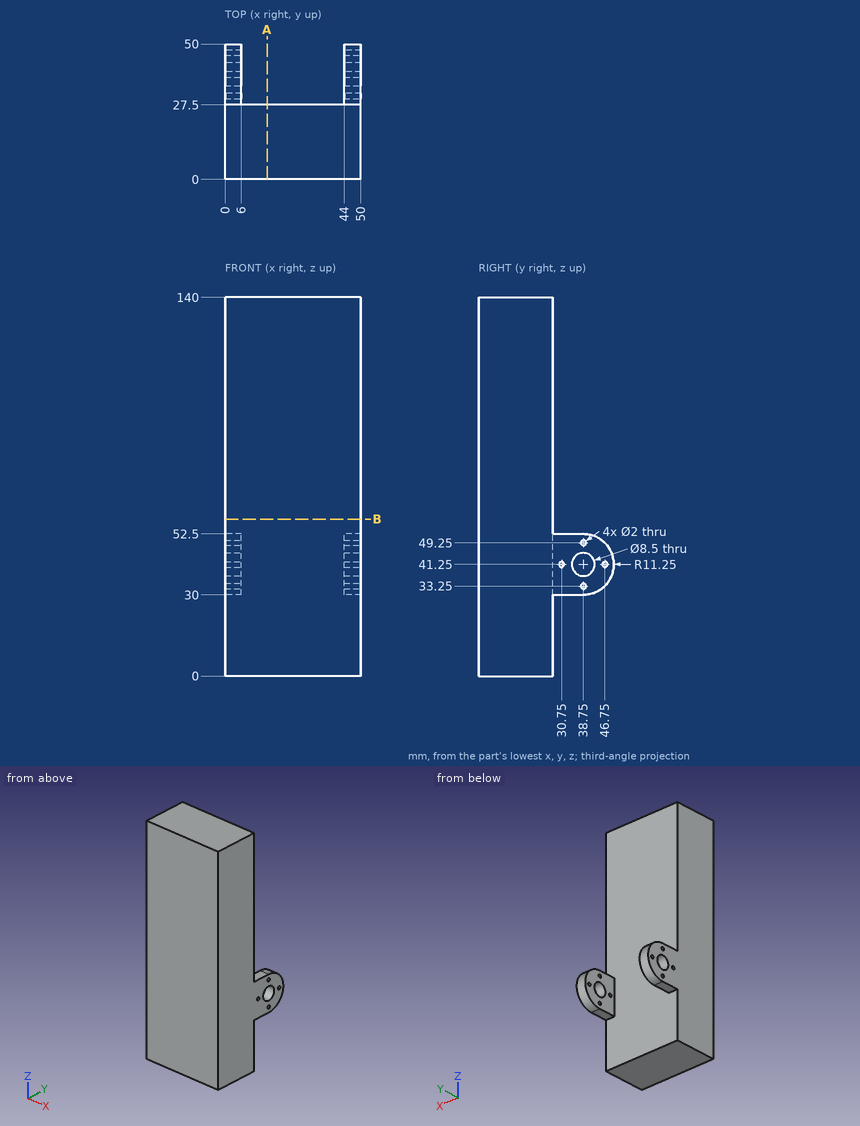
Design review of the part shown in the three views and the two pictorial views. Dimensions are in mm from the part's minimum x, y and z. Round coordinates to 2 decimals unless told otherwise and drop trailing zeros. Loops run counter-clockwise (first coordinate to the right, second up) from the corner with the lowest first, then second, coordinate; pieces in that order, holes last.
(1) Clearance check with flat-ended pins moving along their axes: P1, Ø3, axis at x = 3.5, y = 32.5, coming from the -Z side; P2, Ø3, axis at x = 4, y = 32.5, coming from the +Z side; P3, Ø4, axis at x = 30.5, z = 47.5, coming from the +Y side. State where each tip first meets the part, or that it passes through.
Returned:
P1: stops at z = 30
P2: stops at z = 52.5
P3: stops at y = 27.5
(2) We need section A-A (x = 15.5). Give the boundary of the cut face in (y, z), plus the area to 3 significant figures.
Returned:
outline: (0, 0) - (27.5, 0) - (27.5, 140) - (0, 140) - close
area: 3,850 mm2
(3) Wall thickness on line 1 along Y through (x, z) = (47, 41); line 2 along Z through (x, y) = (2, 38.75); line 3 along Z through (x, y) = (3.7, 30.75): over which ranges is each line inside the solid? List them lowest first.
Returned:
line 1: y = 0 to 29.78, 31.72 to 34.51, 42.99 to 45.78, 47.72 to 50
line 2: z = 30 to 32.25, 34.25 to 37, 45.5 to 48.25, 50.25 to 52.5
line 3: z = 30 to 40.25, 42.25 to 52.5
(4) We need section B-B (z = 58). Give the boundary of the cut face in (x, y).
Returned:
outline: (0, 0) - (50, 0) - (50, 27.5) - (0, 27.5) - close
